Input: dimensioned drawing with shaded views. Units: mm. Origin: part minimum x, y, z. A direction names the side the tool comes from. Give positions to 0.01 mm unless a question says otherwise; leave off trailing zeros. Loops run counter-clockwise (first coordinate to the right, second up) from the corner with the lowest first, then second, coordinate; pieces in that order, holes last. Notation, with made-up numbers: (35.25, -30.75) -> (72.25, -30.75) arc R13 ccw to (72.25, -20.75) -> close; hole circle Ø2 at (8.25, -26.75). An arc over 180 degrees is marked (long way). Answer in a Markdown table with one row per item. Add a question column.
1) Section query D-D (y = 0.5). Return the cut outline in (x, z), plus the area to 3 significant figures.
2) First-contact query: P1, Ø1.2, axis at y = 3.93, z = 15, coming from the +X side; P2, Ø2, axis at y = 2.44, z = 3, coming from the -X side; P3, Ø2, axis at x = 6, y = 4.5, coming from the +Z side. Flat tips, straight axial feed; report the tip coordinate or a pass-through.
3) Line query: line 1 (Y direction, x = 2.5, z = 3) (1 decimal); line 2 (Z direction, x = 1.5, y = 5.75); line 3 (X direction, y = 3.5, z = 9.25). Output: solid intervals per line, ascending. Write a range as from..to.
4) Section query B-B (y = 2.25). Return the cut outline in (x, z).
5) Section query C-C (x = 8). Return the cut outline in (y, z) (1 decimal).
6) Access query for the marked faces 1 and 2. Directions: +Z, -Z, +X, -X, +Y, -Y. A direction counts if a zero-diameter tool reaches every point of the face in a straight line with its end or side. Return the directions, or none.
7) Section query A-A (z = 15). Return the cut outline in (x, y) (1 decimal).
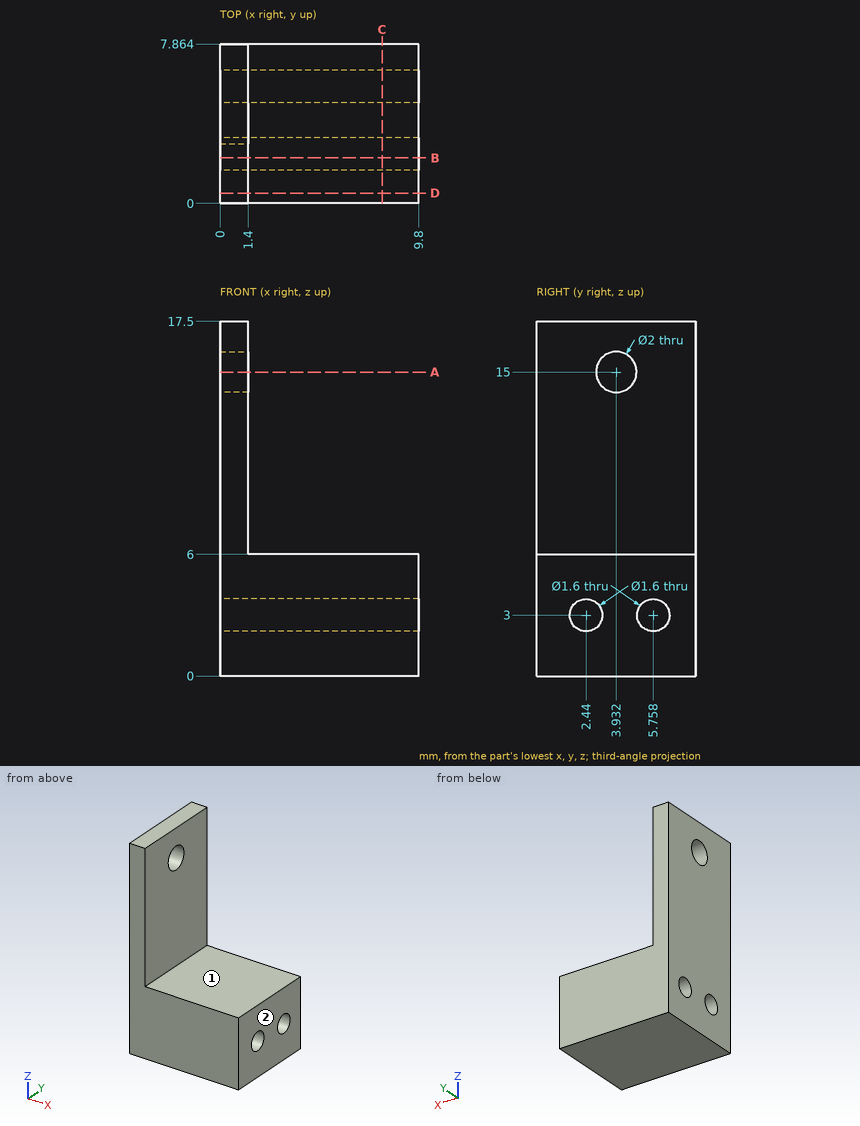
Evaluation:
| question | item | result |
|---|---|---|
| 1 | outline | (0, 0) -> (9.8, 0) -> (9.8, 6) -> (1.4, 6) -> (1.4, 17.5) -> (0, 17.5) -> close |
| 1 | area | 74.9 mm² |
| 2 | P1 | through |
| 2 | P2 | x = 0 |
| 2 | P3 | z = 6 |
| 3 | line 1 | 0..1.6, 3.2..5, 6.6..7.9 |
| 3 | line 2 | 0..2.2, 3.8..6 |
| 3 | line 3 | 0..1.4 |
| 4 | outline | (0, 0) -> (9.8, 0) -> (9.8, 2.22) -> (0, 2.22) -> close; (0, 3.78) -> (9.8, 3.78) -> (9.8, 6) -> (1.4, 6) -> (1.4, 17.5) -> (0, 17.5) -> close |
| 5 | outline | (0, 0) -> (7.9, 0) -> (7.9, 6) -> (0, 6) -> close; hole circle Ø1.6 at (2.4, 3); hole circle Ø1.6 at (5.8, 3) |
| 6 | face 1 | +Z, +X, +Y, -Y |
| 6 | face 2 | +Z, -Z, +X, +Y, -Y |
| 7 | outline | (0, 0) -> (1.4, 0) -> (1.4, 2.9) -> (0, 2.9) -> close; (0, 4.9) -> (1.4, 4.9) -> (1.4, 7.9) -> (0, 7.9) -> close |
